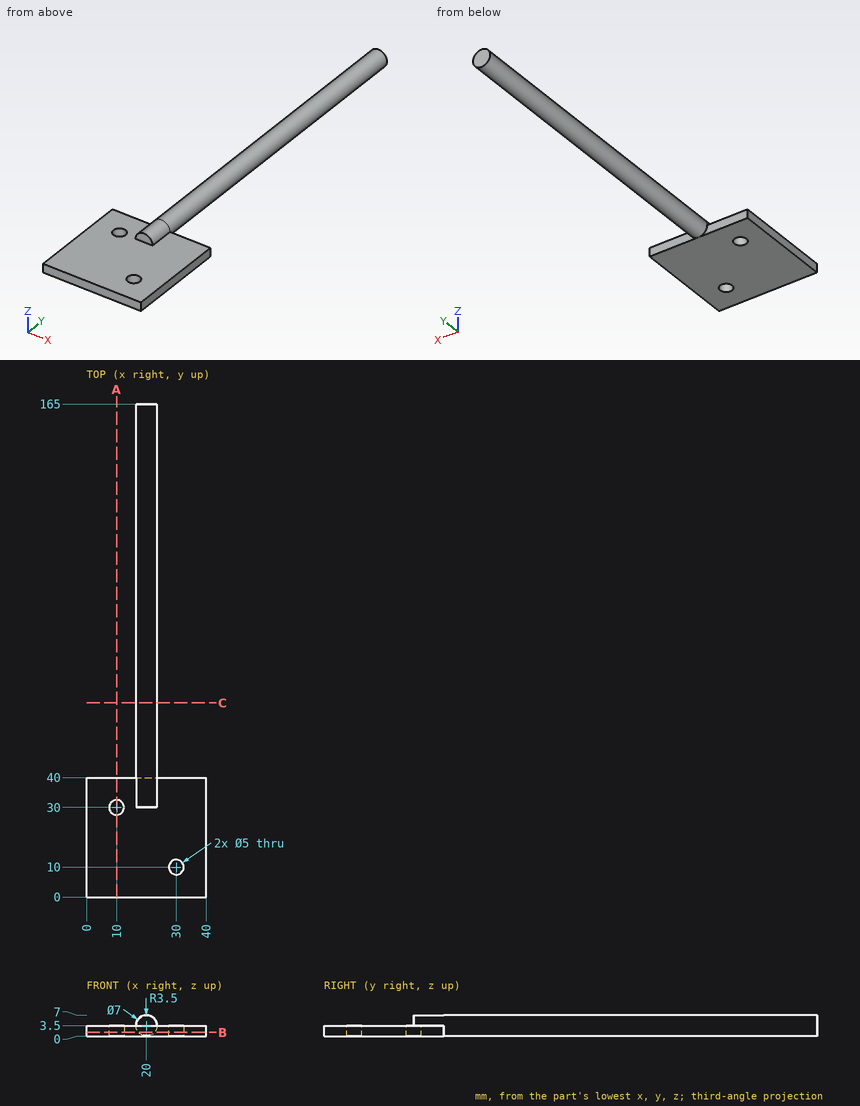
Job drawing, mm, ordinate dimensions from the low corner. One solid piece. Round coordinates to 2 decimals unless told otherwise and drop trailing zeros. Write each loop counter-clockwise with the first axis right and the second up, starting at its lowest first coordinate (ties: lowest second). Pieces come first, ordered by that corner, then holes.
1) Band-saw the part on B-B, the plane z = 1.25. List the corners of the cut face in (x, y).
2) Band-saw the part on C-C, the plane y = 65. List the corners of the cut face in (x, z).
3) Pin check, flat tips, straight feed: pin 1 (6 mm diameter, centred on x = 30, y = 10, fed in from +Z); pin 2 (4 mm diameter, centred on x = 31.5, z = 2.5, fed in from +Y); pin 3 (1.5 mm diameter, centred on x = 17.5, y = 40, fed in from -Z); pin 4 (3 mm diameter, centred on x = 18.5, z = 5.5, fed in from -Y). Stop position of each tip, or through.
4) Drill centre lines: probe 1 along Y at (x, z) = (30, 1.3); probe 2 along Y at (x, z) = (10, 1.7); probe 3 along Z at (x, y) = (32, 38.5). Where is each one in solid material? Low to high.
5) Band-saw the part on A-A, the plane x = 10. List the corners of the cut face in (y, z).
Ans:
1. outline: (0, 0) - (40, 0) - (40, 40) - (22.68, 40) - (22.68, 165) - (17.32, 165) - (17.32, 40) - (0, 40) - close; hole circle Ø5 at (10, 30); hole circle Ø5 at (30, 10)
2. outline: circle Ø7 at (20, 3.5)
3. pin 1: stops at z = 3.5
3. pin 2: stops at y = 40
3. pin 3: stops at z = 0
3. pin 4: stops at y = 30
4. probe 1: y = 0 to 7.5, 12.5 to 40
4. probe 2: y = 0 to 27.5, 32.5 to 40
4. probe 3: z = 0 to 3.5
5. outline: (0, 0) - (27.5, 0) - (27.5, 3.5) - (0, 3.5) - close; (32.5, 0) - (40, 0) - (40, 3.5) - (32.5, 3.5) - close
